Job drawing, mm, ordinate dimensions from the low corner. One solid piece. Give positions to 0.01 mm unless a question says otherwise; leave off trailing zeros. Write each loop counter-clockwise with the first axis right and the second up, starting at its lowest first coordinate (ties: lowest second). Pieces come first, ordered by that corner, then holes. Notation, with made-up numbers: (-12, -21) -> (13, -21) arc R30 ccw to (13, 6) -> close; hole circle Ø5 at (-26, 62.25). An arc over 180 degrees is marked (long way). Put each result on its own line as item: value. Start each with the question number.
Item 1: Slice it at A-A, the plane x = 25. List the corners of the cut face in (y, z) (3 decimals).
Item 2: Slice it at C-C, the plane z = 0.9. List the corners of the cut face in (x, y) (3 decimals), plus the area to 3 significant figures.
Item 3: Slice it at D-D, the plane x = 18. List the corners of the cut face in (y, z) (3 decimals), plus the area to 3 significant figures.
Item 4: Flat gauge pin, fed straight in: pin 1 Ø3 at (x, y) = (18.175, 32.175) entering from +Z. Where does the tip first touch, or does it go through?
Item 5: Drill centre lines: line 1 along Y through (x, z) = (17, 0.5) (3 decimals); line 2 along Y through (x, z) = (18.5, 1.05) (3 decimals). Where is each one in solid material? Low to high.
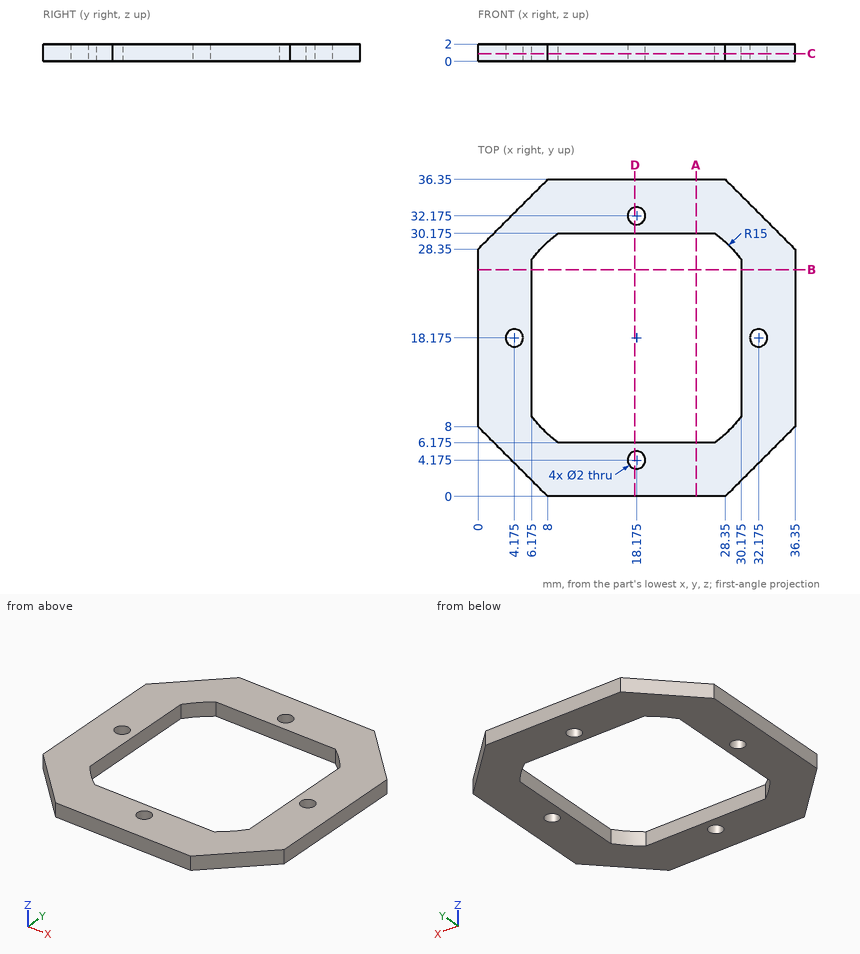
Values follow:
1. outline: (0, 0) -> (6.175, 0) -> (6.175, 2) -> (0, 2) -> close; (30.175, 0) -> (36.35, 0) -> (36.35, 2) -> (30.175, 2) -> close
2. outline: (0, 8) -> (8, 0) -> (28.35, 0) -> (36.35, 8) -> (36.35, 28.35) -> (28.35, 36.35) -> (8, 36.35) -> (0, 28.35) -> close; hole circle Ø2 at (4.175, 18.175); hole (6.175, 9.175) arc R15 ccw to (9.175, 6.175) -> (27.175, 6.175) arc R15 ccw to (30.175, 9.175) -> (30.175, 27.175) arc R15 ccw to (27.175, 30.175) -> (9.175, 30.175) arc R15 ccw to (6.175, 27.175) -> close; hole circle Ø2 at (18.175, 4.175); hole circle Ø2 at (18.175, 32.175); hole circle Ø2 at (32.175, 18.175)
2. area: 621 mm2
3. outline: (0, 0) -> (3.19, 0) -> (3.19, 2) -> (0, 2) -> close; (5.16, 0) -> (6.175, 0) -> (6.175, 2) -> (5.16, 2) -> close; (30.175, 0) -> (31.19, 0) -> (31.19, 2) -> (30.175, 2) -> close; (33.16, 0) -> (36.35, 0) -> (36.35, 2) -> (33.16, 2) -> close
3. area: 16.8 mm2
4. pin 1: z = 2
5. line 1: 0 to 6.175, 30.175 to 36.35
5. line 2: 0 to 3.229, 5.121 to 6.175, 30.175 to 31.229, 33.121 to 36.35
